Input: part model. Units: mm. Frame: model coordinates. Face numbers are marked on the shaded views. A direction names the side the tool comes from. Coordinates: 2 decimals unless noted, no trailing zeros. Loops run counter-clockwise (first coordinate to the right, second up) from the corner with the lowest first, then second, coordinate; pieces in that order, holes last. Notation, with made-up numbers: (-12.5, -1.75) - (44.5, -1.75) arc R29 cw to (44.5, 37.25) - close; hole circle Ø6 at (-3.75, 51). An arc over 180 degrees is marked (long way). Use a Markdown table: item, result. Add a question column.
1. Draft query along X for the marked faces 3, 4 and 5. Return one class per face: released by +X, released by -X, zero draft, split by the parting line, or undercut.
2. Section query C-C on z = -14. Return the cut outline in (x, y), then the cut area to 3 significant figures.
3. Access query for the marked faces 1 and 2. Directions: +Z, -Z, +X, -X, +Y, -Y. A direction counts if a zero-diameter tool reaches every point of the face in a straight line with its end or side. Return the directions, or none.
4. Contact query for flat-ended pins moving along their axis: P1, Ø3, axis at x = 24.5, z = -8.5, coming from the -Y side; P2, Ø3.5, axis at x = 70, y = 2.5, coming from the -Z side. Output: stop coordinate, or through.
5. Section query D-D on z = -7. Return the cut outline in (x, y), then the cut area to 3 significant figures.
6. Section query B-B on x = 69. Return the cut outline in (y, z).
7. Ray query, L1, parallel to X at y = 2.5, z = -13.5; L2, parallel to X at y = 3.75, z = -15; L3, parallel to X at y = 0.75, z = -18. Return the intervals inside material, ascending. Write a range as [from, to].
```python
from build123d import *

# Parameters (mm, degrees)
SKETCH1_W           = 80
SKETCH1_H           = 30
BOSS_EXTRUDE1_DEPTH = 6.5
FILLET1_R           = 15
CUT_EXTRUDE1_REACH  = 87.687
SKETCH2_R           = 2.5
CUT_EXTRUDE2_DEPTH  = 86.686930159
CUT_EXTRUDE3_REACH  = 87.687
CUT_EXTRUDE4_DEPTH  = 86.686930159


with BuildPart() as part:
    # Sketch1 → Boss-Extrude1 (new body)
    with BuildSketch(Plane(origin=(0, 0, 0), x_dir=(1, 0, 0), z_dir=(0, 1, 0))):
        with Locations((40, 15)):
            Rectangle(SKETCH1_W, SKETCH1_H)
    extrude(amount=BOSS_EXTRUDE1_DEPTH)

    # Fillet1
    fillet1_edges = [part.edges().sort_by_distance(p)[0] for p in [
        (0, 3.25, 0),
        (0, 3.25, -30),
    ]]
    fillet(fillet1_edges, radius=FILLET1_R - 0.0001)  # a hair under: the kernel refuses the full size

    # Sketch2 → Cut-Extrude1 (cut, up to next)
    with BuildSketch(Plane(origin=(0, 6.5, 0), x_dir=(1, 0, 0), z_dir=(0, 1, 0)), mode=Mode.PRIVATE) as cut_extrude1_sk1:
        with Locations(Location((15, 15, 0), (0, 0, 270))):
            Circle(SKETCH2_R)
    cut_extrude1_tool1 = extrude(cut_extrude1_sk1.sketch, amount=-CUT_EXTRUDE1_REACH, mode=Mode.PRIVATE) & part.part
    add(cut_extrude1_tool1.solids().sort_by_distance((15, 6.5, -15))[0], mode=Mode.SUBTRACT)

    # Sketch3 → Cut-Extrude2 (cut, through all)
    with BuildSketch(Plane(origin=(0, 6.5, 0), x_dir=(1, 0, 0), z_dir=(0, 1, 0))):
        Polygon((68, 20), (72, 10), (54.850407656, 10), (54.850407656, 23.025538444), (64.248213181, 30), (80, 30), (80, 20), align=None)
    extrude(amount=-CUT_EXTRUDE2_DEPTH, mode=Mode.SUBTRACT)

    # Sketch4 → Cut-Extrude3 (cut, up to next)
    with BuildSketch(Plane(origin=(0, 6.5, 0), x_dir=(1, 0, 0), z_dir=(0, 1, 0)), mode=Mode.PRIVATE) as cut_extrude3_sk1:
        Polygon((80, 20), (80, 0), (72.147195496, 20), align=None)
    cut_extrude3_tool1 = extrude(cut_extrude3_sk1.sketch, amount=-CUT_EXTRUDE3_REACH, mode=Mode.PRIVATE) & part.part
    add(cut_extrude3_tool1.solids().sort_by_distance((77.382398, 6.5, -13.333333))[0], mode=Mode.SUBTRACT)

    # Sketch5 → Cut-Extrude4 (cut, through all)
    with BuildSketch(Plane(origin=(0, 6.5, 0), x_dir=(1, 0, 0), z_dir=(0, 1, 0))):
        Polygon((80, 0), (80, 10), (66.525403502, 0), align=None)
    extrude(amount=-CUT_EXTRUDE4_DEPTH, mode=Mode.SUBTRACT)


solid = part.part
```
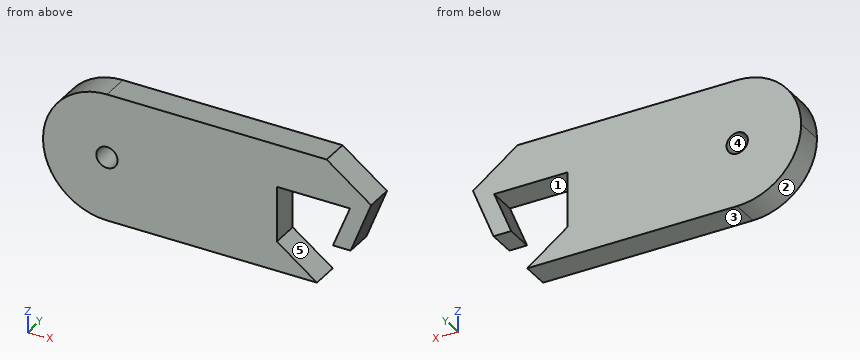
Resolved:
| question | item | result |
|---|---|---|
| 1 | face 3 | zero draft |
| 1 | face 4 | undercut |
| 1 | face 5 | released by +X |
| 2 | outline | (0.03, 0) - (12.71, 0) - (12.71, 6.5) - (0.03, 6.5) - close; (17.29, 0) - (54.85, 0) - (54.85, 6.5) - (17.29, 6.5) - close; (70.4, 0) - (74.5, 0) - (74.5, 6.5) - (70.4, 6.5) - close |
| 2 | area | 353 mm² |
| 3 | face 1 | +Y, -Y |
| 3 | face 2 | -Z, -X, +Y, -Y |
| 4 | P1 | y = 0 |
| 4 | P2 | z = -20 |
| 5 | outline | (2.31, 0) - (75.96, 0) - (75.96, 6.5) - (2.31, 6.5) - close |
| 5 | area | 479 mm² |
| 6 | outline | (0, -20) - (6.5, -20) - (6.5, -17.5) - (0, -17.5) - close; (0, -10) - (6.5, -10) - (6.5, -1.84) - (0, -1.84) - close |
| 7 | L1 | [0.08, 13], [17, 54.85], [70.6, 74.7] |
| 7 | L2 | [0, 12.5], [17.5, 54.85], [70, 74.11] |
| 7 | L3 | [0.3, 54.85], [68.8, 72.93] |
